Geometry check sheet. Reference: the model listing, model coordinates, mm. A direction names the side the tool comes from. Coordinates: 2 decimals unless noted, no trailing zeros. Write each loop counter-clockwise with the first axis right and the second up, starting at its lowest first coordinate (ties: lowest second). Pieces come first, ordered by that corner, then holes. Notation, with made-up numbers: (8, 46) -> (41, 46) arc R7 ccw to (41, 59) -> close; hole circle Ø10 at (5.25, 35.5). An arc over 180 degrees is marked (long way). One line per question, with ' | ' between items.
from build123d import *

# Parameters (mm, degrees)
BOSS_EXTRUDE1_DEPTH = 6.4
SKETCH2_R           = 3
CUT_EXTRUDE1_DEPTH  = 3
SKETCH3_R           = 3
CUT_EXTRUDE2_DEPTH  = 3
CHAMFER1_SIZE       = 1


with BuildPart() as part:
    # Sketch1 → Boss-Extrude1 (new body, symmetric)
    with BuildSketch(Plane.XY):
        with BuildLine():
            Line((3, 0), (27, 0))
            Line((27, 0), (27, 2))
            Line((27, 2), (4.414213562, 2))
            ThreePointArc((4.414213562, 2), (2.707106781, 2.707106781), (2, 4.414213562))
            Line((2, 4.414213562), (2, 27))
            Line((2, 27), (0, 27))
            Line((0, 27), (0, 3))
            ThreePointArc((0, 3), (0.878679656, 0.878679656), (3, 0))
        make_face()
    extrude(amount=BOSS_EXTRUDE1_DEPTH, both=True)

    # Sketch2 → Cut-Extrude1 (cut, through all)
    with BuildSketch(Plane(origin=(0, 2, 0), x_dir=(1, 0, 0), z_dir=(0, 1, 0))):
        with Locations((19.2, 0)):
            Circle(SKETCH2_R)
    extrude(amount=-CUT_EXTRUDE1_DEPTH, mode=Mode.SUBTRACT)

    # Sketch3 → Cut-Extrude2 (cut, through all)
    with BuildSketch(Plane(origin=(2, 0, 0), x_dir=(0, 0, -1), z_dir=(1, 0, 0))):
        with Locations((0, 19.2)):
            Circle(SKETCH3_R)
    extrude(amount=-CUT_EXTRUDE2_DEPTH, mode=Mode.SUBTRACT)

    # Chamfer1
    chamfer1_edges = [part.edges().sort_by_distance(p)[0] for p in [
        (16.2, 2, 0),
        (2, 19.2, 3),
    ]]
    chamfer(chamfer1_edges, length=CHAMFER1_SIZE)


solid = part.part
1. Material ranges on line 1 (Z direction, x = 19.2, y = 0.3); line 2 (X direction, y = 18, z = -5.75), recorded low to high. Write a range as from..to.
Worked answers:
line 1: -6.4..-3, 3..6.4 | line 2: 0..2
2. Mould release check, pull along Z, two halves, no side actions. Record for faces 1 (the face through (21.97, 0.51, 1.15)), 2 (the face through (1, 8, 6.4)), 3 (the face through (2, 13, 0)): released by +Z, released by -Z, zero draft, split by the parting line, or undercut.
Worked answers:
face 1: undercut | face 2: released by +Z | face 3: zero draft
3. Tool access check on faces 4 (the face through (13, 2, 0)), 5 (the face through (27, 1, 0)). Record the directions out of +Z, -Z, +X, -X, +Y, -Y that give a thin tool (end or side, any length) a straight path to the whole face; none if there is none.
Worked answers:
face 4: +Z, -Z, +X, +Y | face 5: +Z, -Z, +X, +Y, -Y
4. Cross-section at A-A on x = 19.2. Record the boundary of the cut face in (y, z).
Worked answers:
outline: (0, -6.4) -> (2, -6.4) -> (2, -4) -> (1, -3) -> (0, -3) -> close; (0, 3) -> (1, 3) -> (2, 4) -> (2, 6.4) -> (0, 6.4) -> close
5. Cross-section at C-C on y = 24. Record the boundary of the cut face in (x, z).
Worked answers:
outline: (0, -6.4) -> (2, -6.4) -> (2, 6.4) -> (0, 6.4) -> close
6. Go/stop test with a flat-tipped pin: P1, Ø4, axis at y = 16.5, z = -2.5, coming from the +X side. Record where the tip stops, or that it passes through.
Worked answers:
P1: x = 2
